```python
from build123d import *

# Parameters (mm, degrees)
F0_W     = 63.5
F0_H     = 38.1
F1_DEPTH = 25.4
F3_DEPTH = 25.4
F5_DEPTH = 25.4


with BuildPart() as f1:
    # F0 (on Front) → F1 (new body)
    with BuildSketch(Plane.XZ):
        with Locations((31.75, 19.05)):
            Rectangle(F0_W, F0_H)
    extrude(amount=F1_DEPTH)

    # F2 (on face) → F3 (cut)
    with BuildSketch(Plane.XZ.offset(25.4)):
        with BuildLine():
            ThreePointArc((0, 27.2450184846), (3.4240390206, 34.6759609794), (10.8549815154, 38.1))
            Line((10.8549815154, 38.1), (0, 38.1))
            Line((0, 38.1), (0, 27.2450184846))
        make_face()
    extrude(amount=-F3_DEPTH, mode=Mode.SUBTRACT)

    # F4 (on face) → F5 (cut)
    with BuildSketch(Plane.XZ.offset(25.4)):
        with BuildLine():
            Line((63.5, 19.05), (63.5, 38.1))
            Line((63.5, 38.1), (32.0302583277, 38.1))
            ThreePointArc((32.0302583277, 38.1), (44.1825704722, 22.6567744591), (63.5, 19.05))
        make_face()
    extrude(amount=-F5_DEPTH, mode=Mode.SUBTRACT)


solid = f1.part
```
Input: part model. Units: mm. Frame: model coordinates. Round coordinates to 2 decimals unless told otherwise and drop trailing zeros. Loops run counter-clockwise (first coordinate to the right, second up) from the corner with the lowest first, then second, coordinate; pieces in that order, holes last. Notation, with made-up numbers: (82, -38) -> (113, -38) arc R24 cw to (113, -11) -> close; hole circle Ø1 at (27, 34.5). An arc over 180 degrees is marked (long way). Use one line per item in the form item = value. Start each with the question number.
Item 1: Section query B-B on x = 5. Return the cut outline in (y, z), then the cut area to 3 significant figures.
Item 2: Material intervals for L1, parallel to Z at x = 58, y = -20; L2, parallel to X at y = -12.5, z = 27; L3, parallel to Z at x = 6, y = -16.5, sorted ascending. Write a range as from..to.
Item 3: Mould query, pull axis X, two halves, no side actions, for faces 1 (the face through (0, -13, 13)), 2 (the face through (43.943, -12.878, 22.804)), 3 (the face through (63.5, -13, 9)). Classes: pulls with the +X half, pulls with the -X half, needs draft (parallel to the pull), parting line crosses it, or undercut.
Item 4: Section query C-C on z = 28. Return the cut outline in (x, y).
Item 5: Section query A-A on y = -21.25. Return the cut outline in (x, z), then the cut area to 3 significant figures.
Item 6: Contact query for flat-ended pins moving along their axis: pin 1 Ø10 at (x, y) = (20, -11.5) entering from -Z; pin 2 Ø1.5 at (x, y) = (55, -2.5) entering from +Z. Output: stop coordinate, or through.
Ans:
q1.outline = (-25.4, 0) -> (0, 0) -> (0, 36) -> (-25.4, 36) -> close
q1.area = 914 mm^2
q2.L1 = 0..18.63
q2.L2 = 0..38.7
q2.L3 = 0..36.63
q3.face_1 = pulls with the -X half
q3.face_2 = undercut
q3.face_3 = pulls with the +X half
q4.outline = (0.08, -25.4) -> (37.77, -25.4) -> (37.77, 0) -> (0.08, 0) -> close
q5.outline = (0, 0) -> (63.5, 0) -> (63.5, 19.05) arc R27.91 cw to (32.03, 38.1) -> (10.85, 38.1) arc R11.81 ccw to (0, 27.25) -> close
q5.area = 1,920 mm^2
q6.pin_1 = 0
q6.pin_2 = 18.97
